Geometry: see drawing. Coordinates: mm, zero at the bounding-box minimum. Coordinates: 2 decimals unless noted, no trailing zeros. Loops run counter-clockwise (first coordinate to the right, second up) from the corner with the lowest first, then second, coordinate; pieces in that order, holes last. Notation, with made-up numbers: (28.5, 54.5) - (63.5, 54.5) arc R19 ccw to (63.5, 64.5) - close; hole circle Ø5 at (68, -19.5). An arc over 180 degrees is marked (long way). Answer in a Markdown table with one row per item.
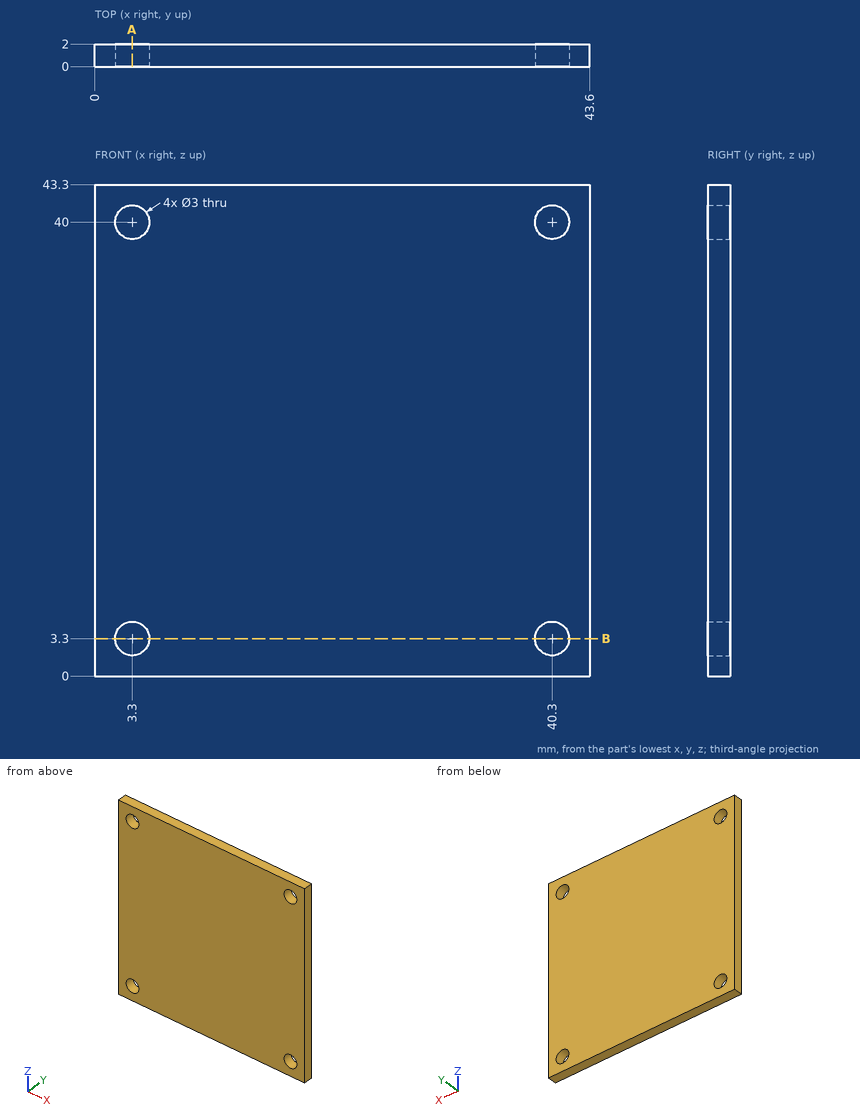
(1) Cut plane A-A on x = 3.3. Output: boundary loops of the cut face in (y, z).
Verdict:
| item | result |
|---|---|
| outline | (0, 0) - (2, 0) - (2, 1.8) - (0, 1.8) - close; (0, 4.8) - (2, 4.8) - (2, 38.5) - (0, 38.5) - close; (0, 41.5) - (2, 41.5) - (2, 43.3) - (0, 43.3) - close |
(2) Cut plane B-B on z = 3.3. Output: boundary loops of the cut face in (x, y).
Verdict:
| item | result |
|---|---|
| outline | (0, 0) - (1.8, 0) - (1.8, 2) - (0, 2) - close; (4.8, 0) - (38.8, 0) - (38.8, 2) - (4.8, 2) - close; (41.8, 0) - (43.6, 0) - (43.6, 2) - (41.8, 2) - close |
(3) First-contact query: pin 1 Ø2.5 at (x, z) = (3.3, 3.3) entering from -Y; pin 2 Ø4 at (x, z) = (3.3, 40) entering from +Y. Flat tips, straight axial feed; report the tip coordinate or a pass-through.
Verdict:
| item | result |
|---|---|
| pin 1 | passes through |
| pin 2 | stops at y = 2 |
(4) Ray query, probe 1 along X at (y, z) = (1.4, 3.3); probe 2 along Z at (x, y) = (40.3, 1.35); probe 3 along Z at (x, y) = (39.5, 1.15). Return the intervals inside material, ascending.
Verdict:
| item | result |
|---|---|
| probe 1 | x = 0 to 1.8, 4.8 to 38.8, 41.8 to 43.6 |
| probe 2 | z = 0 to 1.8, 4.8 to 38.5, 41.5 to 43.3 |
| probe 3 | z = 0 to 2.03, 4.57 to 38.73, 41.27 to 43.3 |
